The listing builds one solid part. Answer for the finished solid, in the listing's coordinates (mm). A direction names the side the tool comes from. Round coordinates to 2 decimals unless told otherwise and drop trailing zeros. Loops run counter-clockwise (first coordinate to the right, second up) from the corner with the lowest first, then second, coordinate; pieces in that order, holes last. Notation, with made-up numbers: (-17.75, 3.25) - (-1.75, 3.25) arc R24 ccw to (-1.75, 41.25) - close; hole circle Ø1 at (56, -28.75). An arc over 180 degrees is marked (long way). One line per item, written item: value.
```python
from build123d import *

# Parameters (mm, degrees)
F0_R     = 4.5
F1_DEPTH = 1


with BuildPart() as f1:
    # F0 (on Front) → F1 (new body)
    with BuildSketch(Plane.XZ):
        with BuildLine():
            Line((-10.607143, 9.214287), (-4.78051, 3.625841))
            ThreePointArc((-4.78051, 3.625841), (3.461877, -4.900552), (-1.819782, 5.717377))
            Line((-1.819782, 5.717377), (-1.819782, 12.266138))
            Line((-1.819782, 12.266138), (-9.146367, 21.857144))
            Line((-9.146367, 21.857144), (-12.878571, 26.742858))
            Line((-12.878571, 26.742858), (-10.607143, 31.285714))
            Line((-10.607143, 31.285714), (-10.607143, 39.000001))
            Line((-10.607143, 39.000001), (-17.892858, 34.500003))
            Line((-17.892858, 34.500003), (-17.892858, 21.857144))
            Line((-17.892858, 21.857144), (-10.607143, 18.214287))
            Line((-10.607143, 18.214287), (-10.607143, 9.214287))
        make_face()
        Circle(F0_R, mode=Mode.SUBTRACT)
    extrude(amount=F1_DEPTH)


solid = f1.part
```
1) For faces 5 (the flat face through (-10.607, -0.5, 13.8)), 6 (the flat face through (-11.76, -0.49, 28.98)), 7 (the cylindrical face through (3.265, -0.493, -5.034)), 8 (the flat face through (-7.735, -0.493, 6.459)), determine the directions among +Z, -Z, +X, -X, +Y, -Y from which every point of the face is accessible in a straight line to the end or side of a thin tool.
Final values:
face 5: -Z, -X, +Y, -Y
face 6: +X, +Y, -Y
face 7: +Y, -Y
face 8: -X, +Y, -Y
2) A cutting plane is placed at D-D on z = 24.5. Give the vertices of the cut face in (x, y).
Final values:
outline: (-17.89, -1) - (-11.17, -1) - (-11.17, 0) - (-17.89, 0) - close
3) Each of these flat-tipped pins is pushed along its axis until it touches: pin 1 Ø0.5 at (y, z) = (-0.5, 34) entering from +X; pin 2 Ø2 at (x, z) = (2, 7.5) entering from -Y. Where does it stop, or does it pass through?
Final values:
pin 1: x = -10.61
pin 2: through
4) A cutting plane is placed at A-A on x = 0. Give the vertices of the cut face in (y, z), and give its area (3 significant figures).
Final values:
outline: (-1, -6) - (0, -6) - (0, -4.5) - (-1, -4.5) - close; (-1, 4.5) - (0, 4.5) - (0, 6) - (-1, 6) - close
area: 3.00 mm2
5) For a pull along Z with two mould halves and no side action, classify faces 1 (the flat face through (-14.2, -0.49, 36.78)), 2 (the flat face through (-14.3, -0.49, 20.06)), 3 (the cylindrical face through (-0.59, -0.49, 4.46)), 4 (the flat face through (-10.607, -0.5, 35.1)) as released by +Z, released by -Z, zero draft, split by the parting line, or undercut.
Final values:
face 1: released by +Z
face 2: released by -Z
face 3: undercut
face 4: zero draft
6) Consider L1, parallel to Z at x = 0, y = -0.75; L2, parallel to X at y = -0.55, z = 10; L3, parallel to Z at x = -12.5, y = -0.05. Determine where each line is inside the solid, lowest interval first.
Final values:
L1: -6 to -4.5, 4.5 to 6
L2: -10.61 to -1.82
L3: 19.16 to 26.25, 27.5 to 37.83
7) A cutting plane is placed at C-C on y = -0.6. Give the vertices of the cut face in (x, z), and give its area (3 significant figures).
Final values:
outline: (-17.89, 21.86) - (-10.61, 18.21) - (-10.61, 9.21) - (-4.78, 3.63) arc R6 ccw (long way) to (-1.82, 5.72) - (-1.82, 12.27) - (-9.15, 21.86) - (-12.88, 26.74) - (-10.61, 31.29) - (-10.61, 39) - (-17.89, 34.5) - close; hole circle Ø9 at (0, 0)
area: 269 mm2
8) A cutting plane is placed at B-B on z = 0. Give the vertices of the cut face in (x, y).
Final values:
outline: (-6, -1) - (-4.5, -1) - (-4.5, 0) - (-6, 0) - close; (4.5, -1) - (6, -1) - (6, 0) - (4.5, 0) - close
